Work out the finished part from the listing and answer in its coordinate system (mm). Face numbers are marked on the shaded views. Give positions to 0.01 mm unless a question says otherwise; leave off trailing zeros. Order: outer loops, then holes, each group sorted by start corner. A loop starts at its lowest first (then second) coordinate and runs counter-clockwise, first axis right, second up. Notation, with made-up numbers: (19, 48.25) -> (37, 48.25) arc R11 cw to (37, 56.25) -> close; hole circle Ø3 at (72.25, 68). An arc over 180 degrees is marked (long way). Use a Markdown table: item, result. Add a question column.
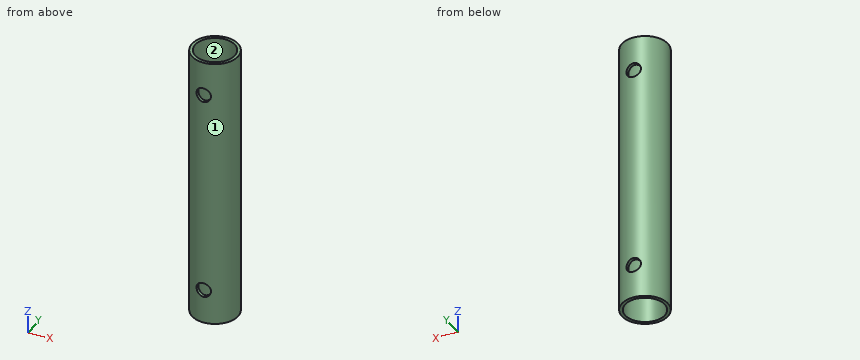
```python
from build123d import *

# Parameters (mm, degrees)
SKETCH1_R               = 6.35
SKETCH1_R_2             = 5.461
EXTRUDE1_DEPTH          = 76.2
SKETCH2_R               = 2
CUT_EXTRUDE1_DEPTH      = 38.1
CUT_EXTRUDE1_DEPTH_BACK = 38.1


with BuildPart() as part:
    # Sketch1 → Extrude1 (new body)
    with BuildSketch(Plane.XY):
        Circle(SKETCH1_R)
        Circle(SKETCH1_R_2, mode=Mode.SUBTRACT)
    extrude(amount=EXTRUDE1_DEPTH)

    # Sketch2 → Cut-Extrude1 (cut, two sides)
    with BuildSketch(Plane(origin=(0, 0, 0), x_dir=(1, 0, 0), z_dir=(0, 1, 0))) as cut_extrude1_sk:
        with Locations((0, -9.525)):
            Circle(SKETCH2_R)
        with Locations((0, -66.675)):
            Circle(SKETCH2_R)
    extrude(amount=CUT_EXTRUDE1_DEPTH, mode=Mode.SUBTRACT)
    extrude(cut_extrude1_sk.sketch, amount=-CUT_EXTRUDE1_DEPTH_BACK, mode=Mode.SUBTRACT)


solid = part.part
```
1) The part is cut by section B-B, the plane y = 0.75. Determine the outline of the cut face in (x, z).
2) Straight lines are drawn through the part: line 1 (Z direction, x = 0, y = -6) (3 decimals); line 2 (Y direction, x = 0, z = 58). For each, find the intervals that lie inside material, in ascending order.
3) The part is cut by section A-A, the plane x = 0. Determine the outline of the cut face in (y, z) (3 decimals).
4) The part is cut by section D-D, the plane z = 46. Determine the outline of the cut face in (x, y).
5) Determine the mould class of the marked faces 1 and 2 for opening direction X: released by +X, released by -X, zero draft, split by the parting line, or undercut.
6) The part is cut by section C-C, the plane x = -3.25. Determine the outline of the cut face in (y, z), then the cut area to 3 significant figures.
7) Flat-ended cylindrical pins translate along their axes: pin 1 (3 mm diameter, centred on y = 2, z = 22, fed in from -X); pin 2 (3.5 mm diameter, centred on x = 0, z = 66.675, fed in from -Y). Find the tip coordinate at first contact, or state that the pin passes through.
A:
| question | item | result |
|---|---|---|
| 1 | outline | (-6.31, 0) -> (-5.41, 0) -> (-5.41, 76.2) -> (-6.31, 76.2) -> close; (5.41, 0) -> (6.31, 0) -> (6.31, 76.2) -> (5.41, 76.2) -> close |
| 2 | line 1 | 0 to 7.525, 11.525 to 64.675, 68.675 to 76.2 |
| 2 | line 2 | -6.35 to -5.46, 5.46 to 6.35 |
| 3 | outline | (-6.35, 0) -> (-5.461, 0) -> (-5.461, 7.525) -> (-6.35, 7.525) -> close; (-6.35, 11.525) -> (-5.461, 11.525) -> (-5.461, 64.675) -> (-6.35, 64.675) -> close; (-6.35, 68.675) -> (-5.461, 68.675) -> (-5.461, 76.2) -> (-6.35, 76.2) -> close; (5.461, 0) -> (6.35, 0) -> (6.35, 7.525) -> (5.461, 7.525) -> close; (5.461, 11.525) -> (6.35, 11.525) -> (6.35, 64.675) -> (5.461, 64.675) -> close; (5.461, 68.675) -> (6.35, 68.675) -> (6.35, 76.2) -> (5.461, 76.2) -> close |
| 4 | outline | circle Ø12.7 at (0, 0); hole circle Ø10.92 at (0, 0) |
| 5 | face 1 | split by the parting line |
| 5 | face 2 | undercut |
| 6 | outline | (-5.46, 0) -> (-4.39, 0) -> (-4.39, 76.2) -> (-5.46, 76.2) -> close; (4.39, 0) -> (5.46, 0) -> (5.46, 76.2) -> (4.39, 76.2) -> close |
| 6 | area | 163 mm^2 |
| 7 | pin 1 | x = -6.33 |
| 7 | pin 2 | through |
